```python
from build123d import *

# Parameters (mm, degrees)
SKETCH1_R           = 2.1
BOSS_EXTRUDE1_DEPTH = 1.5
FILLET1_R           = 2


with BuildPart() as part:
    # Sketch1 → Boss-Extrude1 (new body)
    with BuildSketch(Plane(origin=(0, 0, 0), x_dir=(-1, 0, 0), z_dir=(0, 0, -1))):
        with BuildLine():
            Line((-23.55, 40.8), (-23.55, 35.6))
            Line((-23.55, 35.6), (-28.55, 35.6))
            ThreePointArc((-28.55, 35.6), (-32.15, 32), (-28.55, 28.4))
            Line((-28.55, 28.4), (-23.55, 28.4))
            Line((-23.55, 28.4), (-23.55, -40.8))
            Line((-23.55, -40.8), (23.55, -40.8))
            Line((23.55, -40.8), (23.55, -35.6))
            Line((23.55, -35.6), (28.55, -35.6))
            ThreePointArc((28.55, -35.6), (32.15, -32), (28.55, -28.4))
            Line((28.55, -28.4), (23.55, -28.4))
            Line((23.55, -28.4), (23.55, 40.8))
            Line((23.55, 40.8), (-23.55, 40.8))
        make_face()
        with Locations(Location((-28.55, 32, 0), (0, 0, 180))):
            Circle(SKETCH1_R, mode=Mode.SUBTRACT)
        with Locations((28.55, -32)):
            Circle(SKETCH1_R, mode=Mode.SUBTRACT)
    extrude(amount=BOSS_EXTRUDE1_DEPTH)

    # Fillet1
    fillet1_edges = [part.edges().sort_by_distance(p)[0] for p in [
        (23.55, 40.8, -0.75),
        (23.55, 35.6, -0.75),
        (23.55, 28.4, -0.75),
        (23.55, -40.8, -0.75),
        (-23.55, -40.8, -0.75),
        (-23.55, -35.6, -0.75),
        (-23.55, -28.4, -0.75),
        (-23.55, 40.8, -0.75),
    ]]
    fillet(fillet1_edges, radius=FILLET1_R)


solid = part.part
```
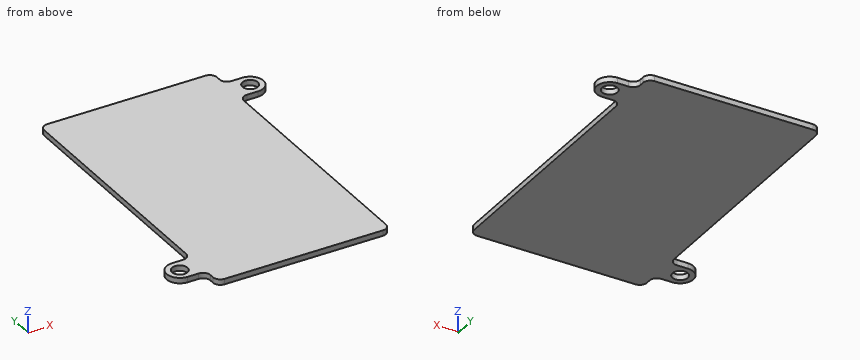
For this review, take the finished solid that the model builds, in its own axes (mm). Coordinates: 2 decimals unless noted, no trailing zeros. Write each loop counter-clockwise with the first axis right and the second up, starting at its lowest first coordinate (ties: lowest second). Pieces come first, ordered by that corner, then holes. Notation, with made-up numbers: (43, 61) - (89, 61) arc R25 cw to (89, 92) - close; hole circle Ø5 at (70.5, 45). An arc over 180 degrees is marked (long way). Answer in a Markdown table with one row per item. Add a question column.
Q1. We need section A-A, the plane z = -0.85. State the section outline as (x, y) points.
Q2. For probe 1 along Y at (x, z) = (28.55, -0.35); probe 2 along Y at (x, z) = (-28.55, -0.8); probe 3 along X at (y, z) = (32, -1.1), list the stretches that pass through material, from the lowest coordinate up.
Q3. We need section C-C, the plane y = 9.5. State the section outline as (x, z) points.
Q4. For P1, Ø0.8, axis at x = -27.5, z = -1, coming from the +Y side; P2, Ø3.5, axis at x = -28.55, y = -32, coming from the +Z side, all flat-tipped, find the tip position at first contact; note any pin that passes through.
Q5. We need section B-B, the plane y = 32. State the section outline as (x, z) points, and give its area (4 significant figures).
Answer list:
| question | item | result |
|---|---|---|
| 1 | outline | (-28.55, -35.6) - (-25.55, -35.6) arc R2 cw to (-23.55, -37.6) - (-23.55, -38.8) arc R2 ccw to (-21.55, -40.8) - (21.55, -40.8) arc R2 ccw to (23.55, -38.8) - (23.55, 26.4) arc R2 cw to (25.55, 28.4) - (28.55, 28.4) arc R3.6 ccw to (28.55, 35.6) - (25.55, 35.6) arc R2 cw to (23.55, 37.6) - (23.55, 38.8) arc R2 ccw to (21.55, 40.8) - (-21.55, 40.8) arc R2 ccw to (-23.55, 38.8) - (-23.55, -26.4) arc R2 cw to (-25.55, -28.4) - (-28.55, -28.4) arc R3.6 ccw to start; hole circle Ø4.2 at (-28.55, -32); hole circle Ø4.2 at (28.55, 32) |
| 2 | probe 1 | y = 28.4 to 29.9, 34.1 to 35.6 |
| 2 | probe 2 | y = -35.6 to -34.1, -29.9 to -28.4 |
| 2 | probe 3 | x = -23.55 to 26.45, 30.65 to 32.15 |
| 3 | outline | (-23.55, -1.5) - (23.55, -1.5) - (23.55, 0) - (-23.55, 0) - close |
| 4 | P1 | stops at y = -28.4 |
| 4 | P2 | passes through |
| 5 | outline | (-23.55, -1.5) - (26.45, -1.5) - (26.45, 0) - (-23.55, 0) - close; (30.65, -1.5) - (32.15, -1.5) - (32.15, 0) - (30.65, 0) - close |
| 5 | area | 77.25 mm2 |
